The listing builds one solid part. Answer for the finished solid, in the listing's coordinates (mm). Round coordinates to 2 decimals unless told otherwise and drop trailing zeros. Loops run counter-clockwise (first coordinate to the right, second up) from the corner with the lowest first, then second, coordinate; pieces in that order, holes last. Notation, with made-up numbers: (-18, -19) -> (40, -19) arc R22 cw to (40, 14) -> close; hole circle Ø4 at (16, -35.75). An arc over 180 degrees is marked (long way). Use a Markdown table: item, result. Add a question column.
Q1. Given pin 1 Ø3.5 at (x, y) = (47.625, -146.05) entering from +Z, flat-ended and moving along its own axis, determine where the tip first touches the part or whether it passes through.
Q2. Section C-C on z = 2.4 is taken. Give the number of separate pieces and of enclosed holes in the cut face, then the cut area to 3 significant figures.
Q3. Consider line 1 (X direction, y = 146.05, z = 2); line 2 (Y direction, x = 99.5, z = 2.8); line 3 (X direction, y = 0.5, z = 1.15). Determine where each line is inside the solid, lowest interval first.
Q4. Section A-A on x = 95.25 is taken. Give the vertices of the cut face in (y, z) (3 decimals).
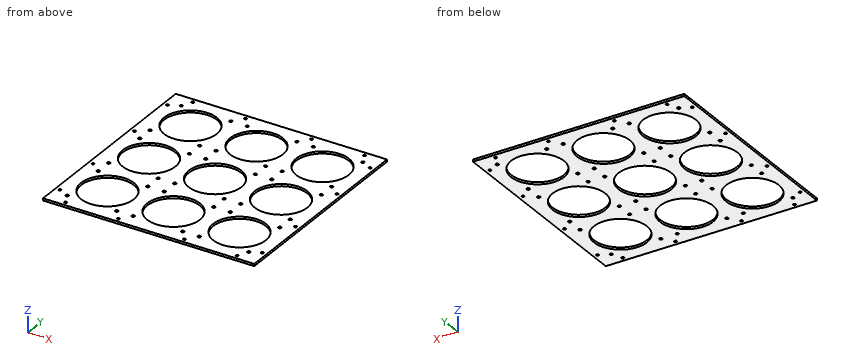
from build123d import *

# Parameters (mm, degrees)
F0_W     = 304.8
F0_H     = 304.8
F0_R     = 2.1463
F0_R_2   = 38.1
F1_DEPTH = 3.175
F2_D     = 3.81


with BuildPart() as f1:
    # F0 (on Top) → F1 (new body)
    with BuildSketch(Plane.XY):
        Rectangle(F0_W, F0_H)
        with Locations((-131.0005, -131.0005)):
            Circle(F0_R, mode=Mode.SUBTRACT)
        with Locations((-95.25, -95.25)):
            Circle(F0_R_2, mode=Mode.SUBTRACT)
        with Locations((-59.4995, -131.0005)):
            Circle(F0_R, mode=Mode.SUBTRACT)
        with Locations((-35.7505, -131.0005)):
            Circle(F0_R, mode=Mode.SUBTRACT)
        with Locations((-131.0005, -59.4995)):
            Circle(F0_R, mode=Mode.SUBTRACT)
        with Locations((-131.0005, -35.7505)):
            Circle(F0_R, mode=Mode.SUBTRACT)
        with Locations((-59.4995, -59.4995)):
            Circle(F0_R, mode=Mode.SUBTRACT)
        with Locations((-35.7505, -59.4995)):
            Circle(F0_R, mode=Mode.SUBTRACT)
        with Locations((-59.4995, -35.7505)):
            Circle(F0_R, mode=Mode.SUBTRACT)
        with Locations((-35.7505, -35.7505)):
            Circle(F0_R, mode=Mode.SUBTRACT)
        with Locations((35.7505, -131.0005)):
            Circle(F0_R, mode=Mode.SUBTRACT)
        with Locations((59.4995, -131.0005)):
            Circle(F0_R, mode=Mode.SUBTRACT)
        with Locations((0, -95.25)):
            Circle(F0_R_2, mode=Mode.SUBTRACT)
        with Locations((131.0005, -131.0005)):
            Circle(F0_R, mode=Mode.SUBTRACT)
        with Locations((95.25, -95.25)):
            Circle(F0_R_2, mode=Mode.SUBTRACT)
        with Locations((35.7505, -59.4995)):
            Circle(F0_R, mode=Mode.SUBTRACT)
        with Locations((59.4995, -59.4995)):
            Circle(F0_R, mode=Mode.SUBTRACT)
        with Locations((35.7505, -35.7505)):
            Circle(F0_R, mode=Mode.SUBTRACT)
        with Locations((59.4995, -35.7505)):
            Circle(F0_R, mode=Mode.SUBTRACT)
        with Locations((131.0005, -59.4995)):
            Circle(F0_R, mode=Mode.SUBTRACT)
        with Locations((131.0005, -35.7505)):
            Circle(F0_R, mode=Mode.SUBTRACT)
        with Locations((-131.0005, 35.7505)):
            Circle(F0_R, mode=Mode.SUBTRACT)
        with Locations((-95.25, 0)):
            Circle(F0_R_2, mode=Mode.SUBTRACT)
        with Locations((-131.0005, 59.4995)):
            Circle(F0_R, mode=Mode.SUBTRACT)
        with Locations((-59.4995, 35.7505)):
            Circle(F0_R, mode=Mode.SUBTRACT)
        with Locations((-35.7505, 35.7505)):
            Circle(F0_R, mode=Mode.SUBTRACT)
        with Locations((-59.4995, 59.4995)):
            Circle(F0_R, mode=Mode.SUBTRACT)
        with Locations((-35.7505, 59.4995)):
            Circle(F0_R, mode=Mode.SUBTRACT)
        with Locations((-95.25, 95.25)):
            Circle(F0_R_2, mode=Mode.SUBTRACT)
        with Locations((-131.0005, 131.0005)):
            Circle(F0_R, mode=Mode.SUBTRACT)
        with Locations((-59.4995, 131.0005)):
            Circle(F0_R, mode=Mode.SUBTRACT)
        with Locations((-35.7505, 131.0005)):
            Circle(F0_R, mode=Mode.SUBTRACT)
        Circle(F0_R_2, mode=Mode.SUBTRACT)
        with Locations((35.7505, 35.7505)):
            Circle(F0_R, mode=Mode.SUBTRACT)
        with Locations((59.4995, 35.7505)):
            Circle(F0_R, mode=Mode.SUBTRACT)
        with Locations((35.7505, 59.4995)):
            Circle(F0_R, mode=Mode.SUBTRACT)
        with Locations((59.4995, 59.4995)):
            Circle(F0_R, mode=Mode.SUBTRACT)
        with Locations((95.25, 0)):
            Circle(F0_R_2, mode=Mode.SUBTRACT)
        with Locations((131.0005, 35.7505)):
            Circle(F0_R, mode=Mode.SUBTRACT)
        with Locations((131.0005, 59.4995)):
            Circle(F0_R, mode=Mode.SUBTRACT)
        with Locations((0, 95.25)):
            Circle(F0_R_2, mode=Mode.SUBTRACT)
        with Locations((35.7505, 131.0005)):
            Circle(F0_R, mode=Mode.SUBTRACT)
        with Locations((59.4995, 131.0005)):
            Circle(F0_R, mode=Mode.SUBTRACT)
        with Locations((95.25, 95.25)):
            Circle(F0_R_2, mode=Mode.SUBTRACT)
        with Locations((131.0005, 131.0005)):
            Circle(F0_R, mode=Mode.SUBTRACT)
    extrude(amount=F1_DEPTH)

    # F2 (through all)
    with Locations(Plane(origin=(0, 0, 0), x_dir=(1, 0, 0), z_dir=(0, 0, -1))):
        with Locations((-146.05, 123.825), (-123.825, 146.05), (123.825, 146.05), (146.05, -123.825), (123.825, -146.05), (-146.05, -123.825), (-123.825, -146.05), (-146.05, 47.625), (-146.05, -47.625), (-47.625, -146.05), (47.625, -146.05), (146.05, -47.625), (146.05, 47.625), (47.625, 146.05), (-47.625, 146.05), (146.05, 123.825)):
            Hole(F2_D / 2)


solid = f1.part
Checked values:
| question | item | result |
|---|---|---|
| 1 | pin 1 | passes through |
| 2 | separate pieces | 1 |
| 2 | enclosed holes | 61 |
| 2 | area | 51,200 mm2 |
| 3 | line 1 | x = -152.4 to -125.73, -121.92 to -49.53, -45.72 to 45.72, 49.53 to 121.92, 125.73 to 152.4 |
| 3 | line 2 | y = -152.4 to -133.11, -57.39 to -37.86, 37.86 to 57.39, 133.11 to 152.4 |
| 3 | line 3 | x = -152.4 to -133.35, -57.15 to -38.1, 38.1 to 57.15, 133.35 to 152.4 |
| 4 | outline | (-152.4, 0) -> (-133.35, 0) -> (-133.35, 3.175) -> (-152.4, 3.175) -> close; (-57.15, 0) -> (-38.1, 0) -> (-38.1, 3.175) -> (-57.15, 3.175) -> close; (38.1, 0) -> (57.15, 0) -> (57.15, 3.175) -> (38.1, 3.175) -> close; (133.35, 0) -> (152.4, 0) -> (152.4, 3.175) -> (133.35, 3.175) -> close |
